Part model, mm, in its own coordinate system. A direction names the side the tool comes from. Round coordinates to 2 decimals unless told otherwise and drop trailing zeros. Order: outer loops, then holes, each group sorted by start corner. A loop starts at its lowest first (then second) coordinate and runs counter-clockwise, first axis right, second up. Notation, with made-up numbers: (59, 18) -> (82, 18) arc R28 cw to (82, 51) -> close; hole circle Ø10 at (57.5, 30.5). An arc over 180 degrees is marked (long way). Use CSV: the item, a comma, the result in double quotes.
```python
from build123d import *

# Parameters (mm, degrees)
SKETCH3_R           = 10
BOSS_EXTRUDE3_DEPTH = 5
SKETCH16_R          = 7.5
BOSS_EXTRUDE7_DEPTH = 50
SKETCH19_R          = 4
CUT_EXTRUDE3_DEPTH  = 50
SKETCH20_R          = 10
BOSS_EXTRUDE8_DEPTH = 5
SKETCH21_W          = 103.138410702
SKETCH21_H          = 76.113402372
BOSS_EXTRUDE9_DEPTH = 70
SCALE1_SCALE        = 2
SKETCH31_R          = 10
CUT_EXTRUDE11_DEPTH = 207.276821406
SKETCH32_W          = 93.138410703
SKETCH32_H          = 55.584947452
CUT_EXTRUDE12_DEPTH = 40


with BuildPart() as part:
    # Sketch3 → Boss-Extrude3 (new body)
    with BuildSketch(Plane.XY):
        Circle(SKETCH3_R)
    extrude(amount=BOSS_EXTRUDE3_DEPTH)

    # Sketch14 → CBORE for M4 Cheese Head Screw1 (revolve, cut)
    with BuildSketch(Plane(origin=(0, 0, 5), x_dir=(0, -1, 0), z_dir=(1, 0, 0))):
        Polygon((0, 0), (0, 8.942065486), (2.4, 7.5), (2.4, 2.6), (4, 2.6), (4, 0.025), (4.025, 0), align=None)
    revolve(axis=Axis((0, 0, 11.35), (0, 0, -1)), mode=Mode.SUBTRACT)

    # Sketch16 → Boss-Extrude7 (add)
    with BuildSketch(Plane.XY.offset(5)):
        Circle(SKETCH16_R)
    extrude(amount=BOSS_EXTRUDE7_DEPTH)

    # Sketch19 → Cut-Extrude3 (cut)
    with BuildSketch(Plane.XY.offset(55)):
        Circle(SKETCH19_R)
    extrude(amount=-CUT_EXTRUDE3_DEPTH, mode=Mode.SUBTRACT)

    # Sketch20 → Boss-Extrude8 (add)
    with BuildSketch(Plane.XY.offset(55)):
        Circle(SKETCH20_R)
    extrude(amount=BOSS_EXTRUDE8_DEPTH)

    # Sketch21 → Boss-Extrude9 (add)
    with BuildSketch(Plane.XY.offset(60)):
        Rectangle(SKETCH21_W, SKETCH21_H)
    extrude(amount=BOSS_EXTRUDE9_DEPTH)


with BuildPart() as part_1:
    # Scale1: scaled about (0, 0, 93.927789278)
    add(part.part.scale(SCALE1_SCALE).moved(Location((0, 0, -93.927789278))))

    # Sketch31 → Cut-Extrude11 (cut, through all)
    with BuildSketch(Plane(origin=(103.138410703, 0, 0), x_dir=(0, 0, -1), z_dir=(1, 0, 0))):
        with BuildLine():
            Line((-30.633863687, 1.766654317), (-26.072210722, 1.766654317))
            Line((-26.072210722, 1.766654317), (-26.072210722, 76.113402371))
            Line((-26.072210722, 76.113402371), (-166.072210722, 76.113402371))
            Line((-166.072210722, 76.113402371), (-166.072210722, -76.113402371))
            Line((-166.072210722, -76.113402371), (-26.072210722, -76.113402371))
            Line((-26.072210722, -76.113402371), (-26.072210722, -1.766654317))
            Line((-26.072210722, -1.766654317), (-30.633863687, -1.766654317))
            Line((-30.633863687, -1.766654317), (-41.414995548, -13.837111886))
            ThreePointArc((-41.414995548, -13.837111886), (-81.657158174, 0), (-41.414995548, 13.837111886))
            Line((-41.414995548, 13.837111886), (-30.633863687, 1.766654317))
        make_face()
        Polygon((-166.072210722, 76.113402371), (-26.072210722, 76.113402371), (-26.072210722, 93.777305116), (-178.92688661, 93.777305116), (-178.92688661, -90.381530622), (-26.072210722, -90.381530622), (-26.072210722, -76.113402371), (-166.072210722, -76.113402371), align=None)
        with Locations((-59.157158174, 0)):
            Circle(SKETCH31_R)
    extrude(amount=-CUT_EXTRUDE11_DEPTH, mode=Mode.SUBTRACT)

    # Sketch32 → Cut-Extrude12 (cut, symmetric)
    with BuildSketch(Plane(origin=(0, 1.766654317, 0), x_dir=(1, 0, 0), z_dir=(0, 1, 0))):
        with Locations((-56.569205352, -53.864684448)):
            Rectangle(SKETCH32_W, SKETCH32_H)
        with Locations((56.569205352, -53.864684448)):
            Rectangle(SKETCH32_W, SKETCH32_H)
    extrude(amount=CUT_EXTRUDE12_DEPTH, both=True, mode=Mode.SUBTRACT)


solid = part_1.part
```
(1) Cut at B-B, the plane z = 56. Give the cut face in (x, y), then the cut area to 3 significant figures.
Reply:
outline,"(-10, -22.28) -> (10, -22.28) -> (10, -9.49) -> (-10, -9.49) -> close; (-10, 9.49) -> (10, 9.49) -> (10, 22.28) -> (-10, 22.28) -> close"
area,"512 mm2"
(2) Drop flat-ended pins along their axis: P1, Ø2.5, axis at x = -0.5, z = 27.5, coming from the -Y side; P2, Ø6, axis at x = 12, z = -55.5, coming from the +Y side; P3, Ø20, axis at x = -8, y = -2.5, coming from the +Z side; P4, Ø1, axis at x = 0, y = 1.5, coming from the +Z side. Give the stop position or say it passes through.
Reply:
P1,"y = -1.77"
P2,"y = 12"
P3,"z = 81.66"
P4,"z = 81.63"
(3) Probe probe 1 along Z at (x, y) = (-8.5, 7.5); probe 2 along X at (y, z) = (-0.5, 7); probe 3 along Y at (x, z) = (0, -85.05). List the from-to ranges inside material, lowest first. Write a range as [from, to].
Reply:
probe 1,"[-93.93, 26.07], [35.75, 52.54], [65.77, 80.37]"
probe 2,"[-14.99, -7.98], [7.98, 14.99]"
probe 3,"[-20, -8], [8, 20]"
(4) Cut at D-D, the plane z = -61. Give the cut face in (x, y).
Reply:
outline,"circle Ø30 at (0, 0); hole circle Ø16 at (0, 0)"
(5) Which spindle directions (+Z, -Z, +X, -X, +Y, -Y) get a long thin tool onto all of the face, cutting with end or side? Do faces 5 (the face through (-10, 0, 48)), 6 (the face through (-4.336, -19.524, -88.998)), 7 (the face through (-14.985, 0.66, -34.628)). Say none if no direction does.
Reply:
face 5,"+Z, -X, +Y, -Y"
face 6,"-Z"
face 7,"none"
(6) Pull direction X, two halves, no side cores. Call faces 1 (the face through (10, 0, 48)), 2 (the face through (-4.336, -19.524, 21.002)), 3 (the face through (0.14, 0.44, 69.147)), 4 (the face through (-4.05, -2.58, -91.49)): released by +X, released by -X, zero draft, split by the parting line, or undercut.
Reply:
face 1,"released by +X"
face 2,"split by the parting line"
face 3,"zero draft"
face 4,"undercut"
